Design review of the part built by this model. Coordinates are the model's own, in mm. A direction names the side the tool comes from. Coordinates: 2 decimals unless noted, no trailing zeros. Write each loop counter-clockwise with the first axis right and the second up, starting at its lowest first coordinate (ties: lowest second). Pieces come first, ordered by that corner, then holes. Notation, with made-up numbers: (25.5, 88) - (39.5, 88) arc R20 ccw to (39.5, 116) - close; hole circle Ø5 at (-1.75, 42). An arc over 180 degrees is marked (long way). Answer as CSV lines item,"result". Start each with the question number.
Q1. For line 1 along Z through (x, y) = (-31, 0); line 2 along X through (y, z) = (7.5, -18.5); line 3 along X through (y, z) = (-16.5, 5.5), list the stretches that pass through material, from the lowest coordinate up. Write a range as [from, to].
Q2. Clearance check with flat-ended pins moving along their axes: pin 1 (3 mm diameter, centred on y = 0, z = 24, fed in from -X); pin 2 (10 mm diameter, centred on y = -11, z = -12, fed in from -X); pin 3 (10 mm diameter, centred on x = -18, y = -17.5, fed in from +Z); pin 4 (3 mm diameter, centred on x = -47, y = 14, fed in from +Z). State where each tip first meets the part, or that it passes through.
Q3. Machinability: for faces 1 (the face through (17, 0, -38)), 2 (the face through (9.5, -2, -30)), 3 (the face through (-31.542, -0.923, 22.226)), which of the approach directions +Z, -Z, +X, -X, +Y, -Y give a long, thin tool a straight path to every point of the face, cutting with its end or side? Answer none if there is none.
Q4. Mouldability with a two-part tool opening along Z and no side actions: class faces 4 (the face through (-56, 0, 4)), 5 (the face through (-28.5, 0, 24)), 6 (the face through (-54.11, 1.08, -4.88)), 7 (the face through (-44.5, -4, -4)) as pulls with the +Z half, pulls with the -Z half, needs draft (parallel to the pull), parting line crosses it, or undercut.
Q5. We need section C-C (x = -26). Write out the cut boundary in (y, z).
Q6. We need section D-D (z = -35). Write out the cut boundary in (x, y), plus the area to 3 significant figures.
Q7. We need section A-A (y = 0). Write out the cut boundary in (x, z), plus the area to 3 significant figures.
Q8. We need section B-B (z = 24). Write out the cut boundary in (x, y), plus the area to 3 significant figures.
from build123d import *

# Parameters (mm, degrees)
F0_R      = 29.5
F1_DEPTH  = 34.5
F2_R      = 18
F3_DEPTH  = 10
F4_R      = 5
F5_DEPTH  = 20
F7_DEPTH  = 25
F8_R      = 5
F9_DEPTH  = 10
F10_R     = 2
F11_DEPTH = 6
F12_W     = 18
F12_H     = 1
F13_DEPTH = 12.5
F14_SIZE  = 0.5


with BuildPart() as f1:
    # F0 (on Right) → F1 (new body, symmetric)
    with BuildSketch(Plane.YZ):
        Circle(F0_R)
    extrude(amount=F1_DEPTH, both=True)

    # F2 (on face) → F3 (join)
    with BuildSketch(Plane(origin=(-34.5, 0, 0), x_dir=(0, -1, 0), z_dir=(-1, 0, 0))):
        Circle(F2_R)
    extrude(amount=F3_DEPTH)

    # F4 (on face) → F5 (join)
    with BuildSketch(Plane(origin=(-44.5, 0, 0), x_dir=(0, -1, 0), z_dir=(-1, 0, 0))):
        Circle(F4_R)
    extrude(amount=F5_DEPTH)

    # F6 (on face) → F7 (join)
    with BuildSketch(Plane.YZ.offset(34.5)):
        with BuildLine():
            Line((29.5, -33.5), (29.5, 0))
            ThreePointArc((29.5, 0), (0, 29.5), (-29.5, 0))
            Line((-29.5, 0), (-29.5, -33.5))
            Line((-29.5, -33.5), (29.5, -33.5))
        make_face()
    extrude(amount=-F7_DEPTH)

    # F8 (on face) → F9 (join)
    with BuildSketch(Plane(origin=(0, 0, -33.5), x_dir=(1, 0, 0), z_dir=(0, 0, -1))):
        with Locations((22, 16)):
            Circle(F8_R)
        with Locations((22, 0)):
            Circle(F8_R)
        with Locations((22, -16)):
            Circle(F8_R)
    extrude(amount=F9_DEPTH)

    # F10 (on face) → F11 (cut)
    with BuildSketch(Plane(origin=(-34.5, 0, 0), x_dir=(0, -1, 0), z_dir=(-1, 0, 0))):
        with Locations((-20.78461, -12)):
            Circle(F10_R)
        with Locations((0, 24)):
            Circle(F10_R)
        with Locations((20.78461, -12)):
            Circle(F10_R)
    extrude(amount=-F11_DEPTH, mode=Mode.SUBTRACT)

    # F12 (on Front) → F13 (cut, symmetric)
    with BuildSketch(Plane.XZ):
        with Locations((-55.5, 4.5)):
            Rectangle(F12_W, F12_H)
    extrude(amount=F13_DEPTH, both=True, mode=Mode.SUBTRACT)

    # F14
    f14_edges = [f1.edges().sort_by_distance(p)[0] for p in [
        (-64.5, 2.236068, -4.472136),
    ]]
    chamfer(f14_edges, length=F14_SIZE)


solid = f1.part
Results list:
1,line 1,"z = [-29.5, 22], [26, 29.5]"
1,line 2,"x = [-34.5, 34.5]"
1,line 3,"x = [-44.5, 34.5]"
2,pin 1,"stops at x = -28.5"
2,pin 2,"stops at x = -44.5"
2,pin 3,"stops at z = 26.72"
2,pin 4,"passes through"
3,face 1,"-Z"
3,face 2,"-Z, -X"
3,face 3,"-X"
4,face 4,"pulls with the +Z half"
4,face 5,"undercut"
4,face 6,"parting line crosses it"
4,face 7,"needs draft"
5,outline,"circle Ø59 at (0, 0)"
6,outline,"circle Ø10 at (22, -16); circle Ø10 at (22, 0); circle Ø10 at (22, 16)"
6,area,"236 mm2"
7,outline,"(-64.5, -4.5) - (-64, -5) - (-44.5, -5) - (-44.5, -18) - (-34.5, -18) - (-34.5, -29.5) - (9.5, -29.5) - (9.5, -33.5) - (17, -33.5) - (17, -43.5) - (27, -43.5) - (27, -33.5) - (34.5, -33.5) - (34.5, 29.5) - (-34.5, 29.5) - (-34.5, 26) - (-28.5, 26) - (-28.5, 22) - (-34.5, 22) - (-34.5, 18) - (-44.5, 18) - (-44.5, 5) - (-46.5, 5) - (-46.5, 4) - (-64.5, 4) - close"
7,area,"4,790 mm2"
8,outline,"(-34.5, -17.15) - (34.5, -17.15) - (34.5, 17.15) - (-34.5, 17.15) - (-34.5, 2) - (-28.5, 2) - (-28.5, -2) - (-34.5, -2) - close"
8,area,"2,340 mm2"
